from build123d import *

# Parameters (mm, degrees)
F0_W        = 1.5
F0_H        = 1.2
F0_W_2      = 0.5
F0_W_3      = 1
F1_DEPTH    = 10
F0_H_2      = 10
F0_H_3      = 0.8
F2_DEPTH    = 5
F3_R        = 0.49999
F4_R        = 0.5
F5_T1_DEPTH = 12.5


# Not quite as in the source:
# - a fillet or chamfer that OpenCascade refuses, or shapes differently, is made with other operations: its cross-section is extruded or revolved along the edge and cut away or added
# - a fillet or chamfer is up to 0.001 mm smaller than in the source, because OpenCascade refuses the exact size


with BuildPart() as f1:
    # F0 (on Front) → F1 (new body)
    with BuildSketch(Plane.XZ):
        Polygon((1, 0.6), (2.5, 0.6), (2.5, -0.6), (1, -0.6), (1, -1.4), (3, -1.4), (3, 1.4), (1, 1.4), align=None)
        Polygon((-2.5, 0.6), (-1, 0.6), (-1, 1.4), (-3, 1.4), (-3, -1.4), (-1, -1.4), (-1, -0.6), (-2.5, -0.6), align=None)
        with Locations((1.75, 0)):
            Rectangle(F0_W, F0_H)
        with Locations((0.75, 0)):
            Rectangle(F0_W_2, F0_H)
        with Locations((-0.75, 0)):
            Rectangle(F0_W_2, F0_H)
        with Locations((-1.75, 0)):
            Rectangle(F0_W, F0_H)
        Rectangle(F0_W_3, F0_H)
    extrude(amount=F1_DEPTH)

    # F0 (on Front) → F2 (join)
    with BuildSketch(Plane.XZ):
        with Locations((0, 5.6)):
            Rectangle(F0_W_3, F0_H_2)
        with Locations((0, -1)):
            Rectangle(F0_W_3, F0_H_3)
    extrude(amount=F2_DEPTH)

    # F3 (radius 0.5 in the source; OpenCascade refuses exactly that, so slightly less here)
    f3_edges = [f1.edges().sort_by_distance(p)[0] for p in [
        (0.5, -2.5, 10.6),
        (-0.5, -2.5, 10.6),
    ]]
    fillet(f3_edges, radius=F3_R)

    # F4
    f4_edges = [f1.edges().sort_by_distance(p)[0] for p in [
        (2, -10, -1.4),
        (3, -10, 0),
        (2, -10, 1.4),
        (1, -10, 1),
        (0, -10, 0.6),
        (-1, -10, 1),
        (-2, -10, 1.4),
        (-3, -10, 0),
        (-2, -10, -1.4),
        (-1, -10, -1),
        (0, -10, -0.6),
        (1, -10, -1),
    ]]
    fillet(f4_edges, radius=F4_R)

    # F5: fillet of radius 0.6 on 8 edges, made by hand

    # F5_s2 → F5_t1 (cut)
    with BuildSketch(Plane.XZ.offset(-1.5)):
        with BuildLine():
            ThreePointArc((-2.4, 1.4), (-2.8242640687, 1.2242640687), (-3, 0.8))
            Line((-3, 0.8), (-3, 1.4))
            Line((-3, 1.4), (-2.4, 1.4))
        make_face()
        with BuildLine():
            ThreePointArc((-1, 0.8), (-1.1757359313, 1.2242640687), (-1.6, 1.4))
            Line((-1.6, 1.4), (-1, 1.4))
            Line((-1, 1.4), (-1, 0.8))
        make_face()
        with BuildLine():
            ThreePointArc((1, 0.8), (1.1757359313, 1.2242640687), (1.6, 1.4))
            Line((1.6, 1.4), (1, 1.4))
            Line((1, 1.4), (1, 0.8))
        make_face()
        with BuildLine():
            ThreePointArc((2.4, 1.4), (2.8242640687, 1.2242640687), (3, 0.8))
            Line((3, 0.8), (3, 1.4))
            Line((3, 1.4), (2.4, 1.4))
        make_face()
        with BuildLine():
            ThreePointArc((-3, -0.8), (-2.8242640687, -1.2242640687), (-2.4, -1.4))
            Line((-2.4, -1.4), (-3, -1.4))
            Line((-3, -1.4), (-3, -0.8))
        make_face()
        with BuildLine():
            ThreePointArc((-1.6, -1.4), (-1.1757359313, -1.2242640687), (-1, -0.8))
            Line((-1, -0.8), (-1, -1.4))
            Line((-1, -1.4), (-1.6, -1.4))
        make_face()
        with BuildLine():
            ThreePointArc((1.6, -1.4), (1.1757359313, -1.2242640687), (1, -0.8))
            Line((1, -0.8), (1, -1.4))
            Line((1, -1.4), (1.6, -1.4))
        make_face()
        with BuildLine():
            ThreePointArc((3, -0.8), (2.8242640687, -1.2242640687), (2.4, -1.4))
            Line((2.4, -1.4), (3, -1.4))
            Line((3, -1.4), (3, -0.8))
        make_face()
    extrude(amount=F5_T1_DEPTH, mode=Mode.SUBTRACT)


solid = f1.part
Input: part model. Units: mm. Frame: model coordinates. Coordinates: 2 decimals unless noted, no trailing zeros. Write each loop counter-clockwise with the first axis right and the second up, starting at its lowest first coordinate (ties: lowest second). Pieces come first, ordered by that corner, then holes. Notation, with made-up numbers: M 70,38.25 L 100,38.25 A5 ccw 100,42.25 Z; hole C 53,79.25 d7. An arc over 180 degrees is marked long. Answer as a JSON object with one key per item and string values. Group by question number.
(1) Contact query for flat-ended pins moving along their axis: P1, Ø4, axis at y = -2, z = 7, coming from the +X side; P2, Ø0.5, axis at x = 0, z = 5.5, coming from the -Y side; P3, Ø2.5, axis at y = -3, z = 7, coming from the -X side. Output: stop coordinate, or through.
(2) Section D-D on z = 4.5. Output: boundary loops of the cut face in (x, y).
(3) Section B-B on x = 0.75. Output: boundary loops of the cut face in (y, z), plus the area to 3 significant figures.
(4) Mould query, pull axis X, two halves, no side actions, for faces 1 (the face through (0, -2, -1.4)), 2 (the face through (-3, -5, 0)), 3 (the face through (0, -6, 0.6)). Classes: pulls with the +X half, pulls with the -X half, needs draft (parallel to the pull), parting line crosses it, or undercut.
(5) Ray query, line 1 along Z through (x, y) = (2.25, -2.75); line 2 along X through (y, z) = (-9, 1); line 3 along Z through (x, y) = (0.5, -6.75). Return the intervals inside material, ascending. Write a range as [from, to].
(6) Section C-C on y = -5.75. Output: boundary loops of the cut face in (x, z), plus the area to 3 significant figures.
Result set:
{
 "1": {"P1": "stops at x = 0.5", "P2": "stops at y = -5", "P3": "stops at x = -0.5"},
 "2": {"outline": "M -0.5,-5 L 0.5,-5 L 0.5,0 L -0.5,0 Z"},
 "3": {"outline": "M -10,-0.1 A0.5 ccw -9.5,-0.6 L 0,-0.6 L 0,0.6 L -9.5,0.6 A0.5 ccw -10,0.1 Z", "area": "11.9 mm2"},
 "4": {"face 1": "needs draft", "face 2": "pulls with the -X half", "face 3": "undercut"},
 "5": {"line 1": "z = [-1.4, 1.4]", "line 2": "x = [-2.97, -1.03], [1.03, 2.97]", "line 3": "z = [-0.6, 0.6]"},
 "6": {"outline": "M -3,-0.8 A0.6 ccw -2.4,-1.4 L -1.6,-1.4 A0.6 ccw -1,-0.8 L -1,-0.6 L 1,-0.6 L 1,-0.8 A0.6 ccw 1.6,-1.4 L 2.4,-1.4 A0.6 ccw 3,-0.8 L 3,0.8 A0.6 ccw 2.4,1.4 L 1.6,1.4 A0.6 ccw 1,0.8 L 1,0.6 L -1,0.6 L -1,0.8 A0.6 ccw -1.6,1.4 L -2.4,1.4 A0.6 ccw -3,0.8 Z", "area": "13.0 mm2"}
}
